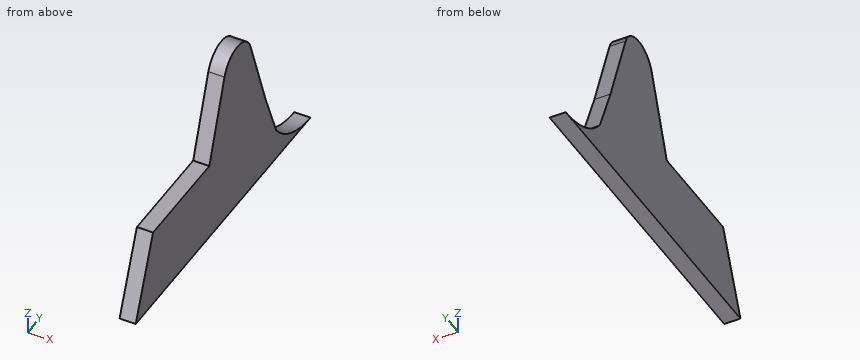
from build123d import *

# Parameters (mm, degrees)
F1_DEPTH = 6.35


with BuildPart() as f1:
    # F0 (on Right) → F1 (new body)
    with BuildSketch(Plane.YZ):
        with BuildLine():
            Line((-53.975, 0), (0, 0))
            Line((0, 0), (53.975, 0))
            Line((53.975, 0), (74.108012, 0))
            ThreePointArc((74.108012, 0), (60.147935, 3.244599), (49.049701, 12.313247))
            Line((49.049701, 12.313247), (41.275, 31.75))
            Line((41.275, 31.75), (30.1625, 63.5))
            ThreePointArc((30.1625, 63.5), (20.6375, 70.257807), (11.1125, 63.5))
            Line((11.1125, 63.5), (0, 31.75))
            Line((0, 31.75), (-41.275, 31.75))
            Line((-41.275, 31.75), (-53.975, 0))
        make_face()
    extrude(amount=F1_DEPTH)


solid = f1.part
Model file for the job. Use its own axes, mm. Round coordinates to 2 decimals unless told otherwise and drop trailing zeros. Order: outer loops, then holes, each group sorted by start corner. A loop starts at its lowest first (then second) coordinate and runs counter-clockwise, first axis right, second up.
(1) Pin check, flat tips, straight feed: pin 1 (3 mm diameter, centred on x = 1.5, z = 31.5, fed in from +Y) (3 decimals); pin 2 (1.5 mm diameter, centred on x = 1.5, z = 50.5, fed in from +Y) (3 decimals); pin 3 (2 mm diameter, centred on x = 4.5, z = 56.5, fed in from +Y); pin 4 (1.5 mm diameter, centred on x = 5, y = -15.5, fed in from -Z). Stop position of each tip, or through.
(2) Band-saw the part on B-B (y = -31). List the corners of the cut face in (x, z), then the cut area to 3 significant figures.
(3) Drill centre lines: line 1 (Z direction, x = 4, y = -20); line 2 (Y direction, x = 0.5, z = 52); line 3 (Y direction, x = 5.25, z = 19) (3 decimals). Where is each one in solid material? Low to high.
(4) Band-saw the part on C-C (z = 58.5). List the corners of the cut face in (x, y), then the cut area to 3 significant figures.
Verdict:
1. pin 1: stops at y = 41.975
1. pin 2: stops at y = 34.975
1. pin 3: stops at y = 32.96
1. pin 4: stops at z = 0
2. outline: (0, 0) - (6.35, 0) - (6.35, 31.75) - (0, 31.75) - close
2. area: 202 mm2
3. line 1: z = 0 to 31.75
3. line 2: y = 7.09 to 34.19
3. line 3: y = -46.375 to 46.375
4. outline: (0, 9.36) - (6.35, 9.36) - (6.35, 31.91) - (0, 31.91) - close
4. area: 143 mm2
